Source: CAD feature listing. Evaluate the final solid. Frame: model axes, mm. Face numbers are marked on the shaded views. A direction names the side the tool comes from. Round coordinates to 2 decimals unless told otherwise and drop trailing zeros. Write each loop counter-clockwise with the first axis right and the second up, starting at its lowest first coordinate (ties: lowest second). Pieces come first, ordered by that corner, then holes. Notation, with made-up numbers: M 28.25,-11 L 68.25,-11 A28 cw 68.25,11 Z; hole C 49.5,27.5 d1. An arc over 180 degrees is marked long. Answer in a Markdown table with one row per item. Add a question column.
Item 1: Set-up query: the marked faces 1, 2, 3, 4 and 5. Return all of +Z, -Z, +X, -X, +Y, -Y with unobstructed straight access to the full face (end or side cutting, diameter ignored); none if empty.
Item 2: Material intervals for probe 1 along Y at (x, z) = (-3.9, 15.3); probe 2 along Y at (x, z) = (-17, 2.4); probe 3 along Y at (x, z) = (-8.75, 21), sorted ascending.
Item 3: Cut plane D-D on x = -17. Return loops of the section in (y, z).
Item 4: Mould query, pull axis Y, two halves, no side actions, for the marked faces 6, 7, 8 and 9. Classes: released by +Y, released by -Y, zero draft, split by the parting line, or undercut.
Item 5: Cut plane C-C on z = 7.3. Return loops of the section in (x, y), and give its area (3 significant figures).
Item 6: Cut plane B-B on x = -9.5. Return loops of the section in (y, z), and give its area (4 significant figures).
Item 7: Cut plane A-A on y = 6. Return loops of the section in (x, z).
Item 8: Contact query for flat-ended pins moving along their axis: pin 1 (2 mm diameter, centred on y = 6.5, z = 15.5, fed in from +X); pin 2 (1.8 mm diameter, centred on x = -4.5, z = 45.5, fed in from +Y); pin 3 (3 mm diameter, centred on y = -6, z = 15.3, fed in from -X); pin 4 (8 mm diameter, centred on x = -14.5, y = -2.5, fed in from -Z). Output: stop coordinate, or through.
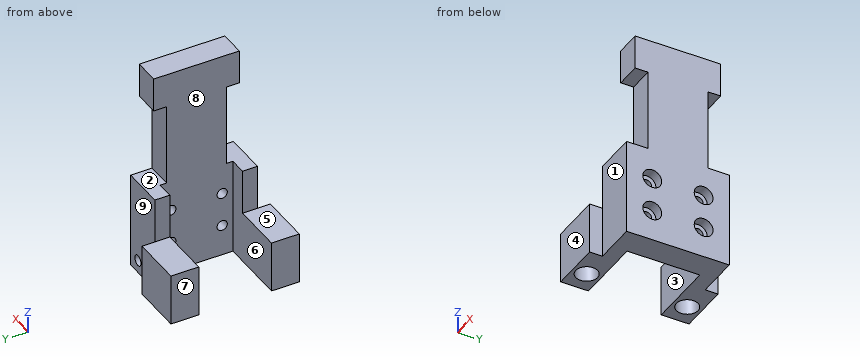
from build123d import *

# Parameters (mm, degrees)
EXTRUDE_1_DEPTH              = 49.6
CUT_EXTRUDE_1_DEPTH          = 31
CUT_EXTRUDE_2_DEPTH          = 49.6
HOLE_WIZARD_M2_1_D           = 2.4
HOLE_WIZARD_M2_1_DEPTH       = 10.1
HOLE_WIZARD_M2_1_CBORE_D     = 4.4
HOLE_WIZARD_M2_1_CBORE_DEPTH = 2.4
HOLE_WIZARD_M2_1_TIP         = 0.721032743
SKETCH_6_R                   = 2.55
CUT_EXTRUDE_3_DEPTH          = 6
HOLE_WIZARD_M3_1_D           = 2.5
HOLE_WIZARD_M3_1_DEPTH       = 7.5
HOLE_WIZARD_M3_1_TIP         = 0.751075774


with BuildPart() as part:
    # 草图1 → 凸台-拉伸1 (new body)
    with BuildSketch(Plane.XY):
        Polygon((-6, 8.5), (-6, -8.5), (-10, -8.5), (-22, -8.5), (-22, -15), (-10, -15), (-10, -12), (0, -12), (0, -10), (0, 10), (0, 12), (-10, 12), (-10, 15), (-22, 15), (-22, 8.5), (-10, 8.5), align=None)
    extrude(amount=EXTRUDE_1_DEPTH)

    # 草图2 → 切除-拉伸1 (cut, through all)
    with BuildSketch(Plane.XZ.offset(15)):
        Polygon((-22, 49.6), (-12.955077182, 49.6), (-6, 49.6), (-6, 22.5), (-10, 22.5), (-10, 12), (-22, 12), align=None)
    extrude(amount=-CUT_EXTRUDE_1_DEPTH, mode=Mode.SUBTRACT)

    # 草图3 → 切除-拉伸2 (cut)
    with BuildSketch(Plane(origin=(0, 0, 0), x_dir=(0, 0, -1), z_dir=(1, 0, 0))):
        Polygon((-22.5, 12), (-41.6, 12), (-49.6, 12), (-49.6, 10), (-41.6, 10), (-41.6, 7), (-22.5, 7), align=None)
        Polygon((-41.6, -12), (-49.6, -12), (-49.6, -10), (-41.6, -10), (-41.6, -7), (-22.5, -7), (-22.5, -12), align=None)
    extrude(amount=-CUT_EXTRUDE_2_DEPTH, mode=Mode.SUBTRACT)

    # M2 六角凹头螺钉的柱形沉头孔1
    with Locations(Plane(origin=(0, 0, 0), x_dir=(0, 0, -1), z_dir=(1, 0, 0))):
        with Locations((-15.3, 6), (-7.3, 6), (-15.3, -6), (-7.3, -6)):
            CounterBoreHole(HOLE_WIZARD_M2_1_D / 2, HOLE_WIZARD_M2_1_CBORE_D / 2, HOLE_WIZARD_M2_1_CBORE_DEPTH, depth=HOLE_WIZARD_M2_1_DEPTH)
            with Locations((0, 0, -(HOLE_WIZARD_M2_1_DEPTH + HOLE_WIZARD_M2_1_TIP / 2))):  # 118° drill point
                Cone(0, HOLE_WIZARD_M2_1_D / 2, HOLE_WIZARD_M2_1_TIP, mode=Mode.SUBTRACT)

    # 草图6 → 切除-拉伸3 (cut)
    with BuildSketch(Plane(origin=(0, 0, 0), x_dir=(-1, 0, 0), z_dir=(0, 0, -1))):
        with Locations((17, -11.75)):
            Circle(SKETCH_6_R)
        with Locations((17, 11.75)):
            Circle(SKETCH_6_R)
    extrude(amount=-CUT_EXTRUDE_3_DEPTH, mode=Mode.SUBTRACT)

    # M3 螺纹孔1
    with Locations(Plane(origin=(0, 12, 0), x_dir=(1, 0, 0), z_dir=(0, 1, 0))):
        with Locations((-3, -3)):
            Hole(HOLE_WIZARD_M3_1_D / 2, depth=HOLE_WIZARD_M3_1_DEPTH)
            with Locations((0, 0, -(HOLE_WIZARD_M3_1_DEPTH + HOLE_WIZARD_M3_1_TIP / 2))):  # 118° drill point
                Cone(0, HOLE_WIZARD_M3_1_D / 2, HOLE_WIZARD_M3_1_TIP, mode=Mode.SUBTRACT)


solid = part.part
Results below:
| question | item | result |
|---|---|---|
| 1 | face 1 | +Z, -Z, +X, -Y |
| 1 | face 2 | +X, -X, +Y |
| 1 | face 3 | +Z, -Z, -X |
| 1 | face 4 | +Z, -Z, +X, -X, -Y |
| 1 | face 5 | +Z, -X, +Y, -Y |
| 2 | probe 1 | -12 to -7.2, -4.8 to 4.8, 7.2 to 12 |
| 2 | probe 2 | -15 to -14.3, -9.2 to -8.5, 8.5 to 9.2, 14.3 to 15 |
| 2 | probe 3 | -12 to -8.5, 8.5 to 12 |
| 3 | outline | M -15,0 L -14.3,0 L -14.3,6 L -9.2,6 L -9.2,0 L -8.5,0 L -8.5,12 L -15,12 Z; M 8.5,0 L 9.2,0 L 9.2,6 L 14.3,6 L 14.3,0 L 15,0 L 15,12 L 8.5,12 Z |
| 4 | face 6 | undercut |
| 4 | face 7 | zero draft |
| 4 | face 8 | undercut |
| 4 | face 9 | released by +Y |
| 5 | outline | M -22,-15 L -10,-15 L -10,-12 L 0,-12 L 0,-8.2 L -2.4,-8.2 L -2.4,-7.2 L -6,-7.2 L -6,-8.5 L -22,-8.5 Z; M -22,8.5 L -6,8.5 L -6,7.2 L -2.4,7.2 L -2.4,8.2 L 0,8.2 L 0,12 L -10,12 L -10,15 L -22,15 Z; M -6,-4.8 L -2.4,-4.8 L -2.4,-3.8 L 0,-3.8 L 0,3.8 L -2.4,3.8 L -2.4,4.8 L -6,4.8 Z |
| 5 | area | 290 mm2 |
| 6 | outline | M -12,0 L -8.5,0 L -8.5,22.5 L -12,22.5 Z; M 8.5,0 L 12,0 L 12,22.5 L 8.5,22.5 Z |
| 6 | area | 157.5 mm2 |
| 7 | outline | M -6,0 L 0,0 L 0,5.1 L -2.4,5.1 L -2.4,6.1 L -6,6.1 Z; M -6,8.5 L -2.4,8.5 L -2.4,9.5 L 0,9.5 L 0,13.1 L -2.4,13.1 L -2.4,14.1 L -6,14.1 Z; M -6,16.5 L -2.4,16.5 L -2.4,17.5 L 0,17.5 L 0,49.6 L -6,49.6 Z; hole C -3,3 d2.5 |
| 8 | pin 1 | x = -2.4 |
| 8 | pin 2 | y = 10 |
| 8 | pin 3 | x = -6 |
| 8 | pin 4 | through |
